Here's how the part is built. I have some questions about the finished solid (model axes, mm). Face numbers are marked on the shaded views. A direction names the side the tool comes from. Give positions to 0.01 mm unless a question says otherwise; leave off trailing zeros. Loops run counter-clockwise (first coordinate to the right, second up) from the corner with the lowest first, then second, coordinate; pieces in that order, holes last. Notation, with made-up numbers: (73, -31.75) - (114, -31.75) arc R19 cw to (114, -15.75) - close; hole circle Ø1 at (51.25, -35). An arc over 180 degrees is marked (long way). Return JSON: item names as keys, results as strings. Group by question number.
(1) If we section it at C-C (z = 10): Please give me the cut outline in (x, y), then the cut area to 3 significant figures.
(2) If we mould it in two halves opening along Y, with no side actions, what happens to the marked faces 4, 5, 6 and 7? For each: released by +Y, released by -Y, zero draft, split by the parting line, or undercut.
(3) On a 3-axis mill with a long thin cutter (end or side, diameter ignored), from which of +Z, -Z, +X, -X, +Y, -Y can I reach the whole of each face in a straight line? I mean the marked faces 1, 2 and 3. Say none if no direction works.
(4) If we section it at A-A (y = 14.25): Please give me the cut outline in (x, z), then the cut area to 3 significant figures.
(5) If we section it at B-B (x = 0): Please give me the cut outline in (y, z).
(6) If we section it at D-D (y = 1.75): Please give me the cut outline in (x, z).
(7) For P1, Ø6.5, axis at x = 0, z = 10, coming from the +Y side; P2, Ø1.5, axis at y = 15.5, z = 13, coming from the -X side, each with a flat end and sliding along its axis, tell me the tip position at first contact or that it passes through.
(8) I need wall thicknesses on probe 1 along Z at (x, y) = (0, 6); probe 2 along Y at (x, z) = (-3, 6.5); probe 3 along Y at (x, z) = (0.25, 15.5) (3 decimals). Which ranges of each line are inside material? Lowest first, please. Write a range as [from, to].
```python
from build123d import *

# Parameters (mm, degrees)
PAD_DEPTH       = 20
FILLET_R        = 1.5
FILLET001_R     = 2
SKETCH001_R     = 2.75
POCKET_DEPTH    = 21.784467
SKETCH002_R     = 5
POCKET001_DEPTH = 6


with BuildPart() as part:
    # Sketch → Pad (new body)
    with BuildSketch(Plane.XY):
        with BuildLine():
            Line((-10, 0), (10, 0))
            Line((10, 0), (10, 8))
            Line((10, 8), (4.582576, 8))
            ThreePointArc((4.582576, 8), (7.626385, 12.87132), (6.480741, 18.5))
            ThreePointArc((5.328024, 21), (5.60069, 19.609971), (6.480741, 18.5))
            ThreePointArc((5.328024, 21), (4.612239, 21.78272), (3.829519, 21.066935))
            ThreePointArc((3.829519, 21.066935), (4.180655, 19.112817), (5.338539, 17.5))
            ThreePointArc((-5.338539, 17.5), (0, 8), (5.338539, 17.5))
            ThreePointArc((-5.338539, 17.5), (-4.180655, 19.112817), (-3.829519, 21.066935))
            ThreePointArc((-3.829519, 21.066935), (-4.612239, 21.78272), (-5.328024, 21))
            ThreePointArc((-6.480741, 18.5), (-5.60069, 19.609971), (-5.328024, 21))
            ThreePointArc((-6.480741, 18.5), (-7.626385, 12.87132), (-4.582576, 8))
            Line((-4.582576, 8), (-10, 8))
            Line((-10, 8), (-10, 0))
        make_face()
    extrude(amount=PAD_DEPTH)

    # Fillet
    fillet_edges = [part.edges().sort_by_distance(p)[0] for p in [
        (4.582576, 8, 10),
        (-4.582576, 8, 10),
    ]]
    fillet(fillet_edges, radius=FILLET_R)

    # Fillet001
    fillet001_edges = [part.edges().sort_by_distance(p)[0] for p in [
        (10, 8, 10),
        (-10, 8, 10),
    ]]
    fillet(fillet001_edges, radius=FILLET001_R)

    # Sketch001 (on Face7 of Fillet001) → Pocket (cut, through all)
    with BuildSketch(Plane.XZ):
        with Locations((0, 10)):
            Circle(SKETCH001_R)
    extrude(amount=-POCKET_DEPTH, mode=Mode.SUBTRACT)

    # Sketch002 (on DatumPlane) → Pocket001 (cut)
    with BuildSketch(Plane.XZ.offset(-10)):
        with Locations((0, 10)):
            Circle(SKETCH002_R)
    extrude(amount=POCKET001_DEPTH, mode=Mode.SUBTRACT)


solid = part.part
```
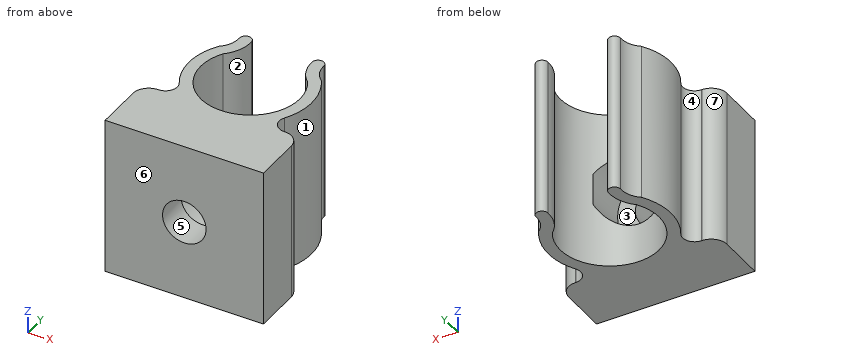
Values:
{
 "1": {"outline": "(-10, 0) - (-2.75, 0) - (-2.75, 4) - (-5, 4) - (-5, 10) - (-4.58, 10) arc R6.25 cw to (-5.34, 17.5) arc R4.5 ccw to (-3.83, 21.07) arc R0.75 ccw to (-5.33, 21) arc R3 cw to (-6.48, 18.5) arc R7.75 ccw to (-6.65, 10.27) arc R1.5 cw to (-7.94, 8) - (-8, 8) arc R2 ccw to (-10, 6) - close; (2.75, 0) - (10, 0) - (10, 6) arc R2 ccw to (8, 8) - (7.94, 8) arc R1.5 cw to (6.65, 10.27) arc R7.75 ccw to (6.48, 18.5) arc R3 cw to (5.33, 21) arc R0.75 ccw to (3.83, 21.07) arc R4.5 ccw to (5.34, 17.5) arc R6.25 cw to (4.58, 10) - (5, 10) - (5, 4) - (2.75, 4) - close", "area": "141 mm2"},
 "2": {"face 4": "undercut", "face 5": "zero draft", "face 6": "released by -Y", "face 7": "released by +Y"},
 "3": {"face 1": "+Z, -Z, +X", "face 2": "+Z, -Z", "face 3": "none"},
 "4": {"outline": "(-7.75, 0) - (-6.25, 0) - (-6.25, 20) - (-7.75, 20) - close; (6.25, 0) - (7.75, 0) - (7.75, 20) - (6.25, 20) - close", "area": "60.0 mm2"},
 "5": {"outline": "(0, 0) - (8, 0) - (8, 5) - (4, 5) - (4, 7.25) - (0, 7.25) - close; (0, 12.75) - (4, 12.75) - (4, 15) - (8, 15) - (8, 20) - (0, 20) - close"},
 "6": {"outline": "(-10, 0) - (10, 0) - (10, 20) - (-10, 20) - close; hole circle Ø5.5 at (0, 10)"},
 "7": {"P1": "y = 4", "P2": "x = -7.73"},
 "8": {"probe 1": "[0, 5], [15, 20]", "probe 2": "[0, 4]", "probe 3": "[0, 8.005]"}
}
